```python
from build123d import *

# Parameters (mm, degrees)
BOSS_EXTRUDE1_DEPTH  = 8.255000001
CUT_EXTRUDE1_DEPTH   = 5.715
BOSS_EXTRUDE2_DEPTH  = 3.175
SKETCH4_W            = 4.572
SKETCH4_H            = 1.143
CUT_EXTRUDE2_DEPTH   = 1.905
SKETCH5_W            = 0.635
SKETCH5_H            = 0.635
BOSS_EXTRUDE3_DEPTH  = 6.096
SKETCH6_W            = 0.635
SKETCH6_H            = 0.635
BOSS_EXTRUDE4_DEPTH  = 6.096
SKETCH7_W            = 0.635
SKETCH7_H            = 1.0668
BOSS_EXTRUDE5_DEPTH  = 1.778
SKETCH8_W            = 0.635
SKETCH8_H            = 1.0668
BOSS_EXTRUDE6_DEPTH  = 1.778
SKETCH9_W            = 0.635
SKETCH9_H            = 0.635
BOSS_EXTRUDE7_DEPTH  = 5.207
SKETCH10_W           = 0.635
SKETCH10_H           = 0.635
BOSS_EXTRUDE8_DEPTH  = 5.207
BOSS_EXTRUDE9_DEPTH  = 1.27
SKETCH12_W           = 1.5875
SKETCH12_H           = 1.778
BOSS_EXTRUDE10_DEPTH = 0.889
SKETCH13_W           = 1.905
SKETCH13_H           = 1.778
BOSS_EXTRUDE11_DEPTH = 0.889
SKETCH14_W           = 1.5875
SKETCH14_H           = 1.778
BOSS_EXTRUDE12_DEPTH = 0.889
FILLET1_R            = 1.27
FILLET2_R            = 1.27
CHAMFER1_SIZE        = 0.508
CHAMFER2_SIZE        = 0.508
DRAFT1_ANGLE         = 45
CHAMFER3_SIZE        = 0.508
FILLET3_R            = 1.016


with BuildPart() as part:
    # Sketch1 → Boss-Extrude1 (new body)
    with BuildSketch(Plane.XY.offset(2.54)):
        Polygon((3.683, 2.286), (-3.683, 2.286), (-3.683, -2.54), (-2.413, -2.54), (-1.651, -3.302), (-1.651, -2.54), (1.651, -2.54), (1.651, -3.302), (2.413, -2.54), (3.683, -2.54), align=None)
    extrude(amount=-BOSS_EXTRUDE1_DEPTH)

    # Sketch2 → Cut-Extrude1 (cut)
    with BuildSketch(Plane.XY.offset(2.54)):
        Polygon((2.667, -1.397), (2.667, 1.27), (1.27, 1.27), (1.27, 2.286000001), (-1.270000001, 2.286000001), (-1.270000001, 1.27), (-2.667, 1.27), (-2.667, -1.397), (-0.508, -1.397), (-0.508, -2.54), (0.508, -2.54), (0.508, -1.397), align=None)
    extrude(amount=-CUT_EXTRUDE1_DEPTH, mode=Mode.SUBTRACT)

    # Sketch3 → Boss-Extrude2 (add)
    with BuildSketch(Plane.XY.offset(2.54)):
        Polygon((0.508, -1.397), (2.667, -1.397), (2.667, 2.921), (-2.667, 2.921), (-2.667, -1.397), (-0.508, -1.397), (-0.508, -2.54), (-1.651, -2.54), (-1.651, -3.302), (-2.413, -2.54), (-3.683, -2.54), (-3.683, 4.064), (3.683, 4.064), (3.683, -2.54), (2.413, -2.54), (1.651, -3.302), (1.651, -2.54), (0.508, -2.54), align=None)
    extrude(amount=BOSS_EXTRUDE2_DEPTH)

    # Sketch4 → Cut-Extrude2 (cut)
    with BuildSketch(Plane(origin=(0, 0, 2.54), x_dir=(-1, 0, 0), z_dir=(0, 0, -1))):
        with Locations((0, 3.4925)):
            Rectangle(SKETCH4_W, SKETCH4_H)
    extrude(amount=-CUT_EXTRUDE2_DEPTH, mode=Mode.SUBTRACT)

    # Sketch5 → Boss-Extrude3 (add)
    with BuildSketch(Plane.XY.offset(-3.175)):
        with Locations((-1.27, -0.0127)):
            Rectangle(SKETCH5_W, SKETCH5_H)
    extrude(amount=BOSS_EXTRUDE3_DEPTH)

    # Sketch6 → Boss-Extrude4 (add)
    with BuildSketch(Plane.XY.offset(-3.175)):
        with Locations((1.27, -0.0127)):
            Rectangle(SKETCH6_W, SKETCH6_H)
    extrude(amount=BOSS_EXTRUDE4_DEPTH)

    # Sketch7 → Boss-Extrude5 (add)
    with BuildSketch(Plane(origin=(0, 0, -5.715000001), x_dir=(-1, 0, 0), z_dir=(0, 0, -1))):
        with Locations((1.27, -0.4826)):
            Rectangle(SKETCH7_W, SKETCH7_H)
    extrude(amount=BOSS_EXTRUDE5_DEPTH)

    # Sketch8 → Boss-Extrude6 (add)
    with BuildSketch(Plane(origin=(0, 0, -5.715000001), x_dir=(-1, 0, 0), z_dir=(0, 0, -1))):
        with Locations((-1.27, -0.4826)):
            Rectangle(SKETCH8_W, SKETCH8_H)
    extrude(amount=BOSS_EXTRUDE6_DEPTH)

    # Sketch9 → Boss-Extrude7 (add)
    with BuildSketch(Plane.XZ.offset(1.016)):
        with Locations((-1.27, -7.1755)):
            Rectangle(SKETCH9_W, SKETCH9_H)
    extrude(amount=BOSS_EXTRUDE7_DEPTH)

    # Sketch10 → Boss-Extrude8 (add)
    with BuildSketch(Plane.XZ.offset(1.016)):
        with Locations((1.27, -7.1755)):
            Rectangle(SKETCH10_W, SKETCH10_H)
    extrude(amount=BOSS_EXTRUDE8_DEPTH)

    # Sketch11 → Boss-Extrude9 (add)
    with BuildSketch(Plane(origin=(0, 0, -6.985), x_dir=(-1, 0, 0), z_dir=(0, 0, -1))):
        Polygon((0.9525, 0.050800001), (1.5875, 0.050800001), (1.5875, -1.016), (3.175, -1.016), (3.175, 1.524), (-3.175, 1.524), (-3.175, -1.016), (-1.5875, -1.016), (-1.5875, 0.050800001), (-0.9525, 0.050800001), (-0.9525, -1.016), (0.9525, -1.016), align=None)
    extrude(amount=-BOSS_EXTRUDE9_DEPTH)

    # Sketch12 → Boss-Extrude10 (add)
    with BuildSketch(Plane(origin=(0, 0, -7.874), x_dir=(-1, 0, 0), z_dir=(0, 0, -1))):
        with Locations((2.38125, -0.127)):
            Rectangle(SKETCH12_W, SKETCH12_H)
    extrude(amount=-BOSS_EXTRUDE10_DEPTH)

    # Sketch13 → Boss-Extrude11 (add)
    with BuildSketch(Plane(origin=(0, 0, -7.874), x_dir=(-1, 0, 0), z_dir=(0, 0, -1))):
        with Locations((0, -0.127)):
            Rectangle(SKETCH13_W, SKETCH13_H)
    extrude(amount=-BOSS_EXTRUDE11_DEPTH)

    # Sketch14 → Boss-Extrude12 (add)
    with BuildSketch(Plane(origin=(0, 0, -7.874), x_dir=(-1, 0, 0), z_dir=(0, 0, -1))):
        with Locations((-2.38125, -0.127)):
            Rectangle(SKETCH14_W, SKETCH14_H)
    extrude(amount=-BOSS_EXTRUDE12_DEPTH)

    # Fillet1
    # the kernel refuses this fillet: 1.27 mm, written as the material it takes off along each edge
    with BuildSketch(Plane(origin=(1.5875, 0.0508, -7.493), x_dir=(0, -1, 0), z_dir=(-1, 0, 0))) as fillet1_piece_1:
        with BuildLine():
            CenterArc((1.016, 1.27), FILLET1_R, 216.869897624, 53.130102376)
            Line((0, 0.508), (0, 0))
            Line((0, 0), (1.016, 0))
        make_face()
    extrude(amount=0.635, mode=Mode.SUBTRACT)

    # Fillet2
    # the kernel refuses this fillet: 1.27 mm, written as the material it takes off along each edge
    with BuildSketch(Plane(origin=(1.5875, 0.0508, -7.493), x_dir=(0, -1, 0), z_dir=(-1, 0, 0))) as fillet2_piece_1_section:
        with BuildLine():
            CenterArc((1.016, 1.27), FILLET2_R, 216.869897624, 53.130102376)
            Line((0, 0.508), (-0.02032, 0.49276))
            ThreePointArc((-0.02032, 0.49276), (-0.0254, 0.254), (-0.0254, 0))
            Line((-0.0254, 0), (0, -0.0254))
            Line((0, -0.0254), (1.016, -0.0254))
            Line((1.016, -0.0254), (1.016, 0))
        make_face()
    fillet2_piece_1 = extrude(amount=3.175, mode=Mode.PRIVATE)
    fillet2_piece_1 = split(fillet2_piece_1, bisect_by=Plane(origin=(0.9525, -0.210671932, -7.36296659), z_dir=(1, 0, 0)), keep=Keep.TOP, mode=Mode.PRIVATE)
    add(fillet2_piece_1, mode=Mode.SUBTRACT)
    with BuildSketch(Plane(origin=(-0.9525, 0.0508, -7.493), x_dir=(0, -1, 0), z_dir=(-1, 0, 0))) as fillet2_piece_2:
        with BuildLine():
            CenterArc((1.016, 1.27), FILLET2_R, 216.869897624, 53.130102376)
            Line((0, 0.508), (-0.02032, 0.49276))
            ThreePointArc((-0.02032, 0.49276), (-0.0254, 0.254), (-0.0254, 0))
            Line((-0.0254, 0), (0, -0.0254))
            Line((0, -0.0254), (1.016, -0.0254))
            Line((1.016, -0.0254), (1.016, 0))
        make_face()
    extrude(amount=0.635, mode=Mode.SUBTRACT)

    # Chamfer1
    chamfer1_edges = [part.edges().sort_by_distance(p)[0] for p in [
        (1.9685, 1.27, 2.54),
    ]]
    chamfer(chamfer1_edges, length=CHAMFER1_SIZE)

    # Chamfer2
    chamfer2_edges = [part.edges().sort_by_distance(p)[0] for p in [
        (-1.9685, 1.27, 2.54),
    ]]
    chamfer(chamfer2_edges, length=CHAMFER2_SIZE)

    # Draft1
    draft1_faces = [part.faces().sort_by_distance(p)[0] for p in [
        (1.651, -2.921, 0),
        (-1.651, -2.921, 0),
    ]]
    draft(draft1_faces, Plane(origin=(-1.651, -2.54, -5.715000001), x_dir=(0, 0, -1), z_dir=(0, -1, 0)), DRAFT1_ANGLE)

    # Chamfer3
    chamfer3_edges = [part.edges().sort_by_distance(p)[0] for p in [
        (-1.5875, -1.397, 5.715),
        (-2.667, 0.762, 5.715),
        (0, 2.921, 5.715),
        (2.667, 0.762, 5.715),
        (1.5875, -1.397, 5.715),
    ]]
    chamfer(chamfer3_edges, length=CHAMFER3_SIZE)

    # Fillet3
    fillet3_edges = [part.edges().sort_by_distance(p)[0] for p in [
        (-2.286, 3.4925, 4.445),
        (2.286, 3.4925, 4.445),
    ]]
    fillet(fillet3_edges, radius=FILLET3_R)


solid = part.part
```
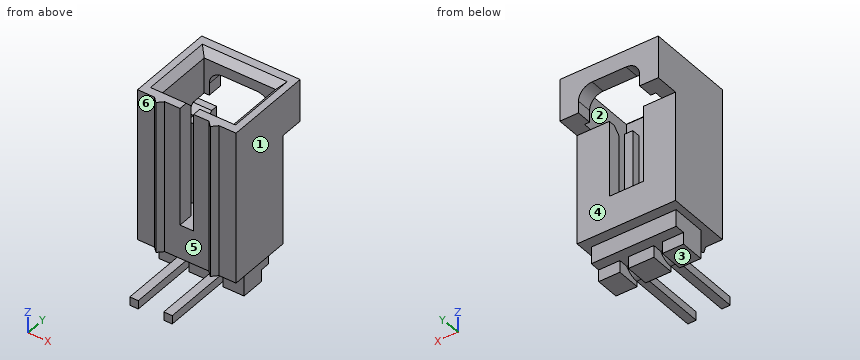
Check sheet for the modelled part. Datum: model origin and axes. Units: mm. Face numbers are marked on the shaded views. A direction names the side the tool comes from. Coordinates: 2 decimals unless noted, no trailing zeros. Loops run counter-clockwise (first coordinate to the right, second up) from the corner with the lowest first, then second, coordinate; pieces in that order, holes last.
1) Sectioned sample at D-D (y = 2). Record the boundary of the cut face in (x, z) (3 decimals).
2) Sectioned sample at B-B (z = 0). Count the separate pieces of the cut face and the enclosed holes in it, and give its area (3 significant figures).
3) Material ranges on probe 1 along X at (y, z) = (0, 0); probe 2 along X at (y, z) = (-2, 0.5); probe 3 along Y at (x, z) = (2.5, -0.25), recorded low to high.
4) Gauge pin test, flat ends, axial feed: pin 1 (4 mm diameter, centred on x = 2, z = 1, fed in from +Y); pin 2 (1.5 mm diameter, centred on x = 1, y = -5, fed in from +Z); pin 3 (1.1 mm diameter, centred on x = -2, z = 1, fed in from +Y); pin 4 (2 mm diameter, centred on x = 1, z = 0.5, fed in from -Y). Record the tip position at first contact, or that the pin passes through.
5) Access from +Z, -Z, +X, -X, +Y, -Y to the whole of each face (thin tool, end or side, straight path). Record for the marked faces 4, 5 and 6.
6) Sectioned sample at C-C (x = 0.25). Record the boundary of the cut face in (y, z) (3 decimals).
7) Release check for a two-part mould opening along X. For the marked faces 1, 2 and 3 record: released by +X, released by -X, zero draft, split by the parting line, or undercut.
8) Sectioned sample at A-A (y = -5). Record the boundary of the cut face in (x, z), and give its area (3 significant figures).
Check sheet entries:
1. outline: (-3.683, -5.715) - (3.683, -5.715) - (3.683, 5.715) - (3.175, 5.715) - (2.667, 5.207) - (2.667, 2.54) - (1.27, 2.54) - (1.27, -3.175) - (-1.27, -3.175) - (-1.27, 2.54) - (-2.667, 2.54) - (-2.667, 5.207) - (-3.175, 5.715) - (-3.683, 5.715) - close
2. separate pieces: 4
2. enclosed holes: 0
2. area: 18.7 mm2
3. probe 1: x = -3.68 to -2.67, -1.59 to -0.95, 0.95 to 1.59, 2.67 to 3.68
3. probe 2: x = -3.68 to -0.51, 0.51 to 3.68
3. probe 3: y = -2.54 to -1.4, 1.27 to 2.29
4. pin 1: stops at y = 4.06
4. pin 2: stops at z = -6.86
4. pin 3: stops at y = 2.29
4. pin 4: stops at y = -2.89
5. face 4: -Z, +X, -X, +Y
5. face 5: +Z, -Y
5. face 6: +Z, -Z, -X, -Y
6. outline: (-2.54, -5.715) - (-1.016, -5.715) - (-1.016, -7.874) - (0.762, -7.874) - (0.762, -6.985) - (1.524, -6.985) - (1.524, -5.715) - (2.286, -5.715) - (2.286, -3.175) - (-2.54, -3.175) - close; (2.921, 4.445) - (4.064, 4.445) - (4.064, 5.715) - (3.429, 5.715) - (2.921, 5.207) - close
7. face 1: released by +X
7. face 2: undercut
7. face 3: zero draft
8. outline: (-1.59, -7.49) - (-0.95, -7.49) - (-0.95, -6.86) - (-1.59, -6.86) - close; (0.95, -7.49) - (1.59, -7.49) - (1.59, -6.86) - (0.95, -6.86) - close
8. area: 0.806 mm2
